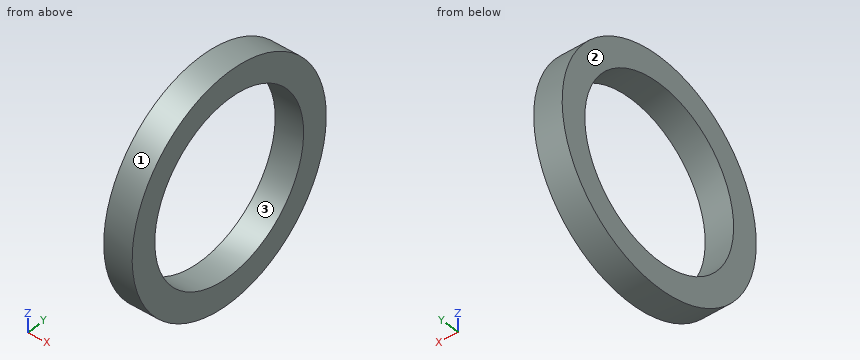
```python
from build123d import *

# Parameters (mm, degrees)
F0_R     = 6
F1_DEPTH = 1.5
F2_R     = 4.6
F3_DEPTH = 1.501
F4_ANGLE = 90
F6_ANGLE = 90


with BuildPart() as f1:
    # F0 (on Front) → F1 (new body)
    with BuildSketch(Plane.XZ):
        Circle(F0_R)
    extrude(amount=-F1_DEPTH)

    # F2 (on face) → F3 (cut, through all)
    with BuildSketch(Plane.XZ):
        Circle(F2_R)
    extrude(amount=-F3_DEPTH, mode=Mode.SUBTRACT)


with BuildPart() as f1_1:
    # F4: moved
    add(f1.part.rotate(Axis((0, 0, 0), (0, -1, 0)), F4_ANGLE))


with BuildPart() as f1_2:
    # F6: moved
    add(f1_1.part.rotate(Axis((0, 0, 0.289831), (0, 0, 1)), F6_ANGLE))


solid = f1_2.part
```
Can you work these out from the model? Positions are in its coordinate system, mm. Face numbers are marked on the shaded views. Give positions to 0.01 mm unless a question says otherwise; leave off trailing zeros. Order: outer loops, then holes, each group sorted by start corner. A loop starts at its lowest first (then second) coordinate and runs counter-clockwise, first axis right, second up. Notation, with made-up numbers: M 11.5,73.25 L 65.5,73.25 A26 ccw 65.5,102.25 Z; hole C 19,69.25 d7. An arc over 180 degrees is marked long. One line per item, written item: value.
1) Please list where these lines run through material, in increasing order: line 1 along Y through (x, z) = (-0.9, 0); line 2 along Z through (x, y) = (-1.05, -4); line 3 along Y through (x, z) = (-0.6, -3.5).
Answer sheet:
line 1: y = -6 to -4.6, 4.6 to 6
line 2: z = -4.47 to -2.27, 2.27 to 4.47
line 3: y = -4.87 to -2.98, 2.98 to 4.87
2) I want a section at A-A, the plane y = 0. List the corners of the cut face in (x, z) for me, plus the area to 3 significant figures.
Answer sheet:
outline: M -1.5,-6 L 0,-6 L 0,-4.6 L -1.5,-4.6 Z; M -1.5,4.6 L 0,4.6 L 0,6 L -1.5,6 Z
area: 4.20 mm^2
3) We'd pull the mould along Z, two halves only. Please class the marked faces 1, 2 and 3: released by +Z, released by -Z, zero draft, split by the parting line, or undercut.
Answer sheet:
face 1: split by the parting line
face 2: zero draft
face 3: undercut
4) I want a section at C-C, the plane x = -0.9. List the corners of the cut face in (y, z) for me.
Answer sheet:
outline: C 0,0 d12; hole C 0,0 d9.2
5) I want a section at D-D, the plane z = 5.25. List the corners of the cut face in (x, y) for me.
Answer sheet:
outline: M -1.5,-2.9 L 0,-2.9 L 0,2.9 L -1.5,2.9 Z
